Verification items for this drawing (mm, ordinates from the low corner). Give positions to 0.01 mm unless a question says otherwise; leave off trailing zeros. Loops run counter-clockwise (first coordinate to the right, second up) from the corner with the lowest first, then second, coordinate; pieces in that order, holes last. Notation, with made-up numbers: (-15, -38) -> (-7, -38) arc R21 ccw to (-7, -25) -> close; hole circle Ø9 at (87.25, 4.25). An arc over 180 degrees is marked (long way). Answer in a Markdown table with one row per item. Add a question column.
Q1. Section check C-C on y = 11. Enter the section's corners in (x, z).
Q2. Section check B-B on y = 3.75. Enter the section's corners in (x, z), and give its area (3 significant figures).
Q3. Material ranges on probe 1 along Y at (x, z) = (6, 31); probe 2 along X at (y, z) = (5.75, 19.5) (1 decimal); probe 3 along X at (y, z) = (8.25, 14), recorded low to high.
Q4. Gauge pin test, flat end, axial feed: P1, Ø3, axis at y = 11, z = 28, coming from the -X side. Record the tip position at first contact, or that the pin passes through.
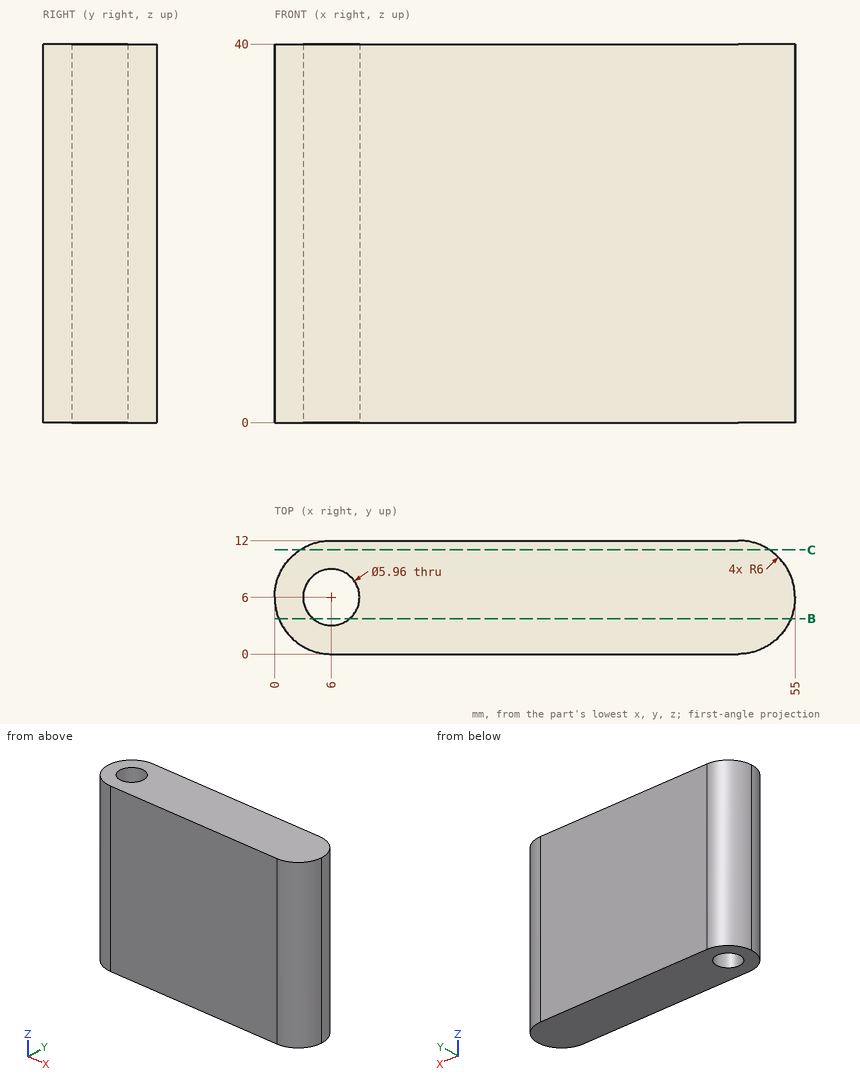
Taken from the geometry:
| question | item | result |
|---|---|---|
| 1 | outline | (2.68, 0) -> (52.32, 0) -> (52.32, 40) -> (2.68, 40) -> close |
| 2 | outline | (0.44, 0) -> (4.05, 0) -> (4.05, 40) -> (0.44, 40) -> close; (7.95, 0) -> (54.56, 0) -> (54.56, 40) -> (7.95, 40) -> close |
| 2 | area | 2,010 mm² |
| 3 | probe 1 | y = 0 to 3.02, 8.98 to 12 |
| 3 | probe 2 | x = 0 to 3, 9 to 55 |
| 3 | probe 3 | x = 0.44 to 4.05, 7.95 to 54.56 |
| 4 | P1 | stops at x = 1.13 |
